Part print with two shaded views. Sizes in mm from the minimum x, y, z corner. Give positions to 0.01 mm unless a question says otherwise; leave off trailing zeros. Write each loop counter-clockwise with the first axis right and the second up, starting at its lowest first coordinate (ties: lowest second). Pieces come first, ordered by that corner, then holes. Notation, with made-up numbers: (15.25, 66.5) -> (71.25, 66.5) arc R26 ccw to (71.25, 90.5) -> close; hole circle Ø1 at (35.25, 2). An arc over 180 degrees is marked (long way). Answer as a JSON object with one key per item and string values.
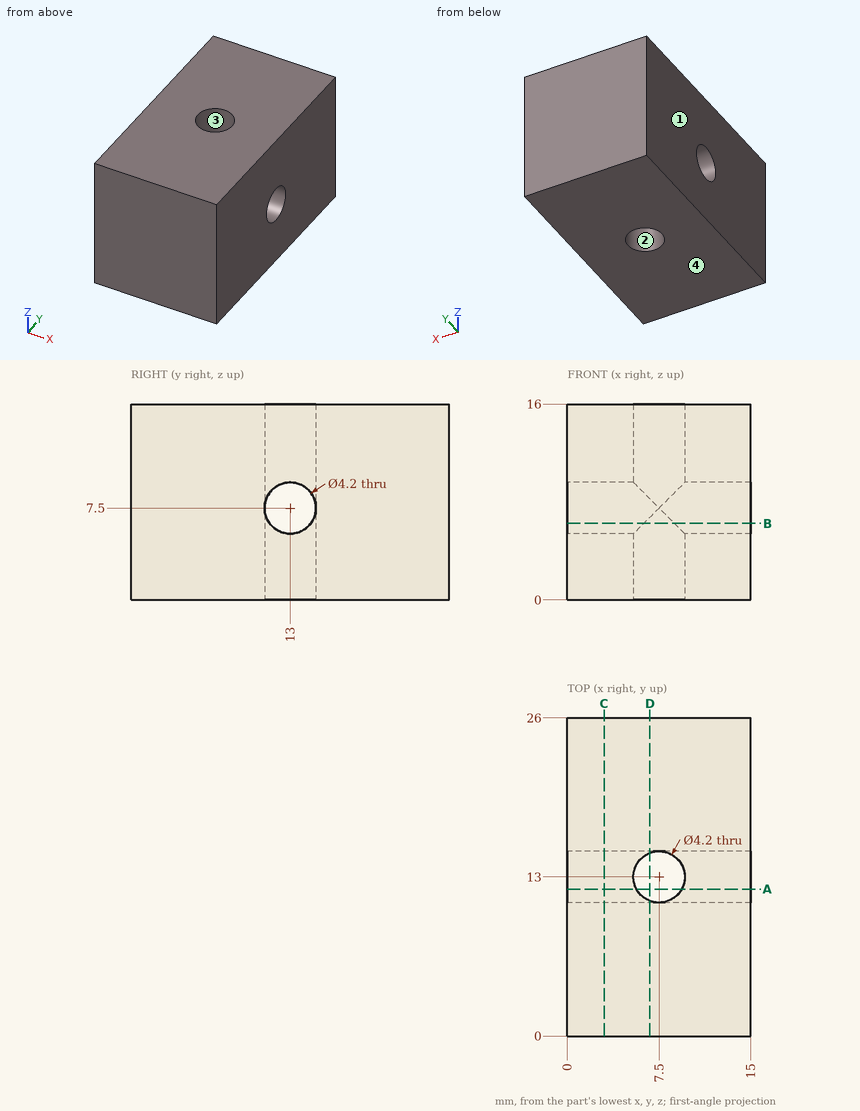
1) Wall check: probe 1 along Y at (x, z) = (7.5, 11.75); probe 2 along X at (y, z) = (13, 12.5); probe 3 along Z at (x, y) = (12.75, 13). Give the ranges that are in metal, low to high.
Model answer:
{"probe 1": "y = 0 to 10.9, 15.1 to 26", "probe 2": "x = 0 to 5.4, 9.6 to 15", "probe 3": "z = 0 to 5.4, 9.6 to 16"}
2) Slice it at B-B (z = 6.25). List the corners of the cut face in (x, y).
Model answer:
{"outline": "(0, 0) -> (15, 0) -> (15, 11.31) -> (8.75, 11.31) arc R2.1 cw to (6.25, 11.31) -> (0, 11.31) -> close; (0, 14.69) -> (6.25, 14.69) arc R2.1 cw to (8.75, 14.69) -> (15, 14.69) -> (15, 26) -> (0, 26) -> close"}
3) Mould opens along X. For the marked faces 1, 2, 3 and 4 say: released by +X, released by -X, zero draft, split by the parting line, or undercut.
Model answer:
{"face 1": "released by -X", "face 2": "undercut", "face 3": "undercut", "face 4": "zero draft"}
4) Slice it at C-C (x = 3). List the corners of the cut face in (y, z).
Model answer:
{"outline": "(0, 0) -> (26, 0) -> (26, 16) -> (0, 16) -> close; hole circle Ø4.2 at (13, 7.5)"}
5) Slice it at A-A (y = 12). List the corners of the cut face in (x, z).
Model answer:
{"outline": "(0, 0) -> (5.65, 0) -> (5.65, 5.65) -> (0, 5.65) -> close; (0, 9.35) -> (5.65, 9.35) -> (5.65, 16) -> (0, 16) -> close; (9.35, 0) -> (15, 0) -> (15, 5.65) -> (9.35, 5.65) -> close; (9.35, 9.35) -> (15, 9.35) -> (15, 16) -> (9.35, 16) -> close"}
6) Slice it at D-D (x = 6.75). List the corners of the cut face in (y, z).
Model answer:
{"outline": "(0, 0) -> (11.04, 0) -> (11.04, 6.75) arc R2.1 cw to (11.04, 8.25) -> (11.04, 16) -> (0, 16) -> close; (14.96, 0) -> (26, 0) -> (26, 16) -> (14.96, 16) -> (14.96, 8.25) arc R2.1 cw to (14.96, 6.75) -> close"}
